from build123d import *

# Parameters (mm, degrees)
SKETCH1_R           = 4
BOSS_EXTRUDE1_DEPTH = 287.5
SKETCH2_R           = 4
BOSS_EXTRUDE2_DEPTH = 45
SKETCH3_R           = 4
CUT_EXTRUDE1_DEPTH  = 105
SKETCH4_R           = 4
BOSS_EXTRUDE3_DEPTH = 68.5


with BuildPart() as part:
    # Sketch1 → Boss-Extrude1 (new body)
    with BuildSketch(Plane.XY):
        Circle(SKETCH1_R)
    extrude(amount=BOSS_EXTRUDE1_DEPTH)

    # Sketch2 → Boss-Extrude2 (add)
    with BuildSketch(Plane.XY.offset(287.5)):
        Circle(SKETCH2_R)
    extrude(amount=BOSS_EXTRUDE2_DEPTH)

    # Sketch3 → Cut-Extrude1 (cut)
    with BuildSketch(Plane(origin=(0, 0, 0), x_dir=(-1, 0, 0), z_dir=(0, 0, -1))):
        Circle(SKETCH3_R)
    extrude(amount=-CUT_EXTRUDE1_DEPTH, mode=Mode.SUBTRACT)

    # Sketch4 → Boss-Extrude3 (add)
    with BuildSketch(Plane(origin=(0, 0, 105), x_dir=(-1, 0, 0), z_dir=(0, 0, -1))):
        Circle(SKETCH4_R)
    extrude(amount=BOSS_EXTRUDE3_DEPTH)


solid = part.part
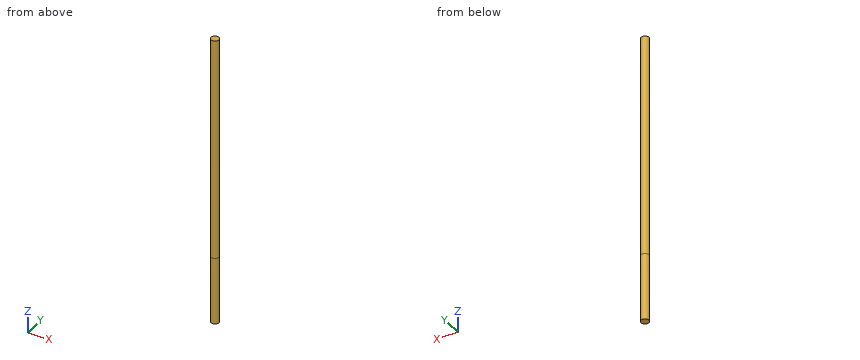
Design review of the part built by this model. Coordinates are the model's own, in mm. Round coordinates to 2 decimals unless told otherwise and drop trailing zeros. Write each loop counter-clockwise with the first axis right and the second up, starting at its lowest first coordinate (ties: lowest second). Pieces come first, ordered by that corner, then holes. Notation, with made-up numbers: (78.25, -36) - (136.25, -36) arc R7 cw to (136.25, -23) - close; hole circle Ø3 at (27, 11). An arc over 180 degrees is marked (long way). Use a Markdown table: item, result. Add a question column.
1. We need section A-A (z = 88). State the section outline as (x, y) points.
2. We need section C-C (y = 2.25). State the section outline as (x, z) points.
3. Clearance check with flat-ended pins moving along their axes: pin 1 (4 mm diameter, centred on y = 1, z = 76.5, fed in from -X); pin 2 (3 mm diameter, centred on x = -2, z = 224.5, fed in from +Y); pin 3 (1 mm diameter, centred on x = 3, z = 234, fed in from +Y). State where each tip first meets the part, or that it passes through.
4. Wall thickness on probe 1 along Y at (x, z) = (0.5, 238); probe 2 along Y at (x, z) = (-3.5, 314); probe 3 along X at (y, z) = (-0.25, 235): over which ranges is each line inside the solid? List them lowest first.
5. We need section B-B (x = -2.5). State the section outline as (y, z) points.
Output:
| question | item | result |
|---|---|---|
| 1 | outline | circle Ø8 at (0, 0) |
| 2 | outline | (-3.31, 36.5) - (3.31, 36.5) - (3.31, 332.5) - (-3.31, 332.5) - close |
| 3 | pin 1 | stops at x = -4 |
| 3 | pin 2 | stops at y = 3.97 |
| 3 | pin 3 | stops at y = 3.12 |
| 4 | probe 1 | y = -3.97 to 3.97 |
| 4 | probe 2 | y = -1.94 to 1.94 |
| 4 | probe 3 | x = -3.99 to 3.99 |
| 5 | outline | (-3.12, 36.5) - (3.12, 36.5) - (3.12, 332.5) - (-3.12, 332.5) - close |
